```python
from build123d import *

# Parameters (mm, degrees)
EXTRUDE_1_DEPTH     = 5.5
CHAMFER_1_SIZE      = 0.6
CHAMFER_1_SIZE2     = 1.039230485
SKETCH_2_W          = 35
SKETCH_2_H          = 15
CUT_EXTRUDE_1_DEPTH = 4.5
FILLET_1_R          = 3
SKETCH_3_R          = 1
EXTRUDE_2_DEPTH     = 1.5


with BuildPart() as part:
    # Эскиз1 → Бобышка-Вытянуть1 (new body)
    with BuildSketch(Plane.XY):
        Polygon((19.75, 0), (-19.75, 0), (-19.75, 33), (-17.75, 35), (-14.75, 35), (-14.75, 46.5), (14.75, 46.5), (14.75, 35), (17.75, 35), (19.75, 33), align=None)
    extrude(amount=EXTRUDE_1_DEPTH)

    # Фаска1
    chamfer_1_edges = [part.edges().sort_by_distance(p)[0] for p in [
        (0, 46.5, 0),
        (-14.75, 46.5, 2.75),
        (14.75, 46.5, 2.75),
        (0, 46.5, 5.5),
    ]]
    chamfer_1_side = [part.faces().sort_by_distance(p)[0] for p in [
        (0, 46.5, 2.75),
    ]]
    chamfer(chamfer_1_edges, length=CHAMFER_1_SIZE, length2=CHAMFER_1_SIZE2, reference=chamfer_1_side[0])

    # Эскиз2 → Вырез-Вытянуть1 (cut)
    with BuildSketch(Plane.XY.offset(5.5)):
        with Locations((0, 17.5)):
            Rectangle(SKETCH_2_W, SKETCH_2_H)
    extrude(amount=-CUT_EXTRUDE_1_DEPTH, mode=Mode.SUBTRACT)

    # Скругление1
    fillet_1_edges = [part.edges().sort_by_distance(p)[0] for p in [
        (17.5, 10, 3.25),
        (17.5, 25, 3.25),
        (-17.5, 25, 3.25),
        (-17.5, 10, 3.25),
    ]]
    fillet(fillet_1_edges, radius=FILLET_1_R)

    # Эскиз3 → Бобышка-Вытянуть2 (add)
    with BuildSketch(Plane.XZ):
        with Locations(Location((0, 2.5, 0), (0, 0, 90))):
            Circle(SKETCH_3_R)
    extrude(amount=EXTRUDE_2_DEPTH)


solid = part.part
```
Geometry check sheet. Reference: the model listing, model coordinates, mm. A direction names the side the tool comes from. Coordinates: 2 decimals unless noted, no trailing zeros. Order: outer loops, then holes, each group sorted by start corner. A loop starts at its lowest first (then second) coordinate and runs counter-clockwise, first axis right, second up.
Item 1: Mould release check, pull along Y, two halves, no side actions. Record for faces 4 (the flat face through (-0.206, 45.973, 5.204)), 5 (the flat face through (0, 23, 0)), 6 (the cylindrical face through (16.6, 24.14, 3.22)): released by +Y, released by -Y, zero draft, split by the parting line, or undercut.
Item 2: Depth check by flat-ended pin: pin 1 (12 mm diameter, centred on x = -14, y = 23.5, fed in from -Z); pin 2 (8 mm diameter, centred on x = 4.5, y = 18, fed in from +Z); pin 3 (1.3 mm diameter, centred on x = -4.5, z = 2.5, fed in from -Y); pin 4 (0.9 mm diameter, centred on x = 16, z = 4, fed in from +Y). Enter the tip coordinate at first touch or a pass-through.
Item 3: Section check C-C (y = 21.5). Enter the section's corners in (x, z).
Item 4: Section check A-A (z = 4.3). Enter the section's corners in (x, y).
Item 5: Section check B-B (x = 0). Enter the section's corners in (y, z).
Item 6: Section check D-D (x = -5.5). Enter the section's corners in (y, z).
Item 7: Scan lines: line 1 along Y through (x, z) = (2, 1.75); line 2 along X through (y, z) = (20, 2.6); line 3 along Y through (x, z) = (10.5, 5.2). Record each from-to range of solid material in increasing order.
Item 8: Tool access check on faces 1 (the cylindrical face through (0, -0.7, 1.5)), 2 (the cylindrical face through (-16.64, 24.1, 3.22)), 3 (the flat face through (-14.75, 40, 3)). Record the directions out of +Z, -Z, +X, -X, +Y, -Y that give a thin tool (end or side, any length) a straight path to the whole face; none if there is none.
Check sheet entries:
1. face 4: released by +Y
1. face 5: zero draft
1. face 6: undercut
2. pin 1: stops at z = 0
2. pin 2: stops at z = 1
2. pin 3: stops at y = 0
2. pin 4: stops at y = 35
3. outline: (-19.75, 0) - (19.75, 0) - (19.75, 5.5) - (17.5, 5.5) - (17.5, 1) - (-17.5, 1) - (-17.5, 5.5) - (-19.75, 5.5) - close
4. outline: (-19.75, 0) - (19.75, 0) - (19.75, 33) - (17.75, 35) - (14.75, 35) - (14.75, 45.46) - (14.15, 46.5) - (-14.15, 46.5) - (-14.75, 45.46) - (-14.75, 35) - (-17.75, 35) - (-19.75, 33) - close; hole (-17.5, 13) arc R3 ccw to (-14.5, 10) - (14.5, 10) arc R3 ccw to (17.5, 13) - (17.5, 22) arc R3 ccw to (14.5, 25) - (-14.5, 25) arc R3 ccw to (-17.5, 22) - close
5. outline: (-1.5, 1.5) - (0, 1.5) - (0, 0) - (45.46, 0) - (46.5, 0.6) - (46.5, 4.9) - (45.46, 5.5) - (25, 5.5) - (25, 1) - (10, 1) - (10, 5.5) - (0, 5.5) - (0, 3.5) - (-1.5, 3.5) - close
6. outline: (0, 0) - (45.46, 0) - (46.5, 0.6) - (46.5, 4.9) - (45.46, 5.5) - (25, 5.5) - (25, 1) - (10, 1) - (10, 5.5) - (0, 5.5) - close
7. line 1: y = 0 to 10, 25 to 46.5
7. line 2: x = -19.75 to -17.5, 17.5 to 19.75
7. line 3: y = 0 to 10, 25 to 45.98
8. face 1: -Y
8. face 2: +Z
8. face 3: +Z, -Z, -X, +Y
